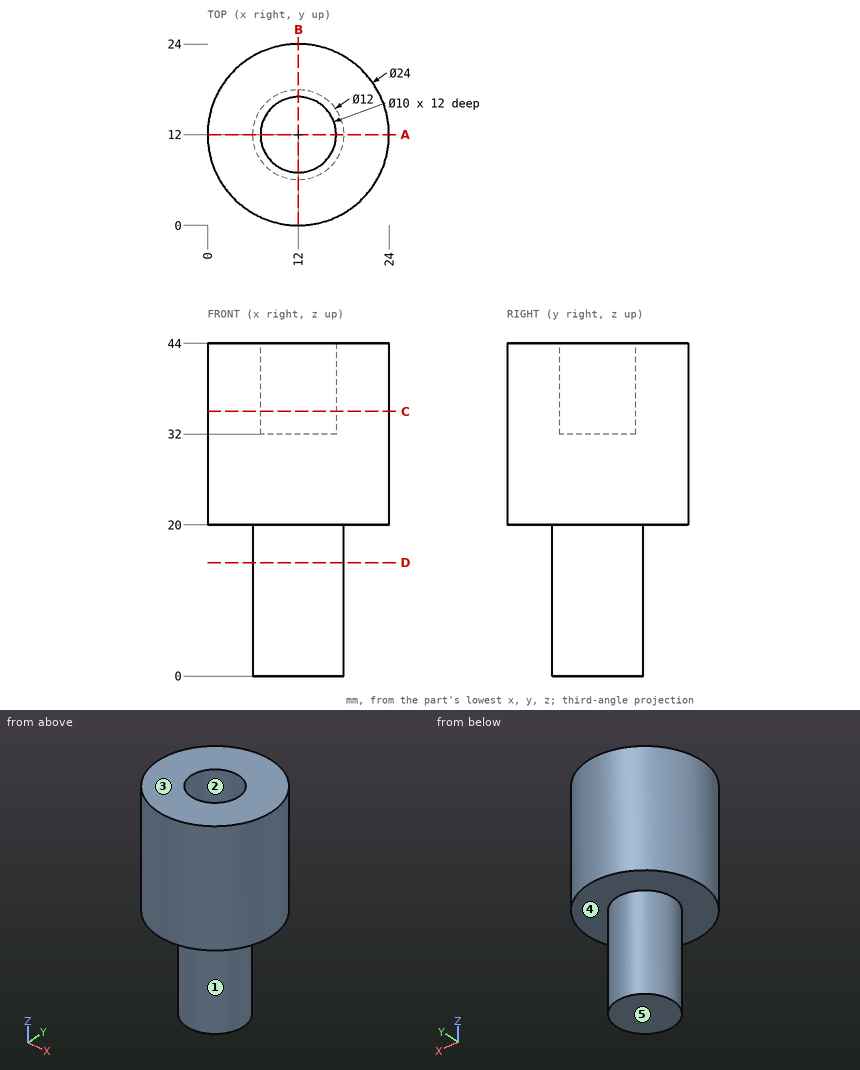
Design review of the part shown in the three views and the two pictorial views. Dimensions are in mm from the part's minimum x, y and z. A direction names the side the tool comes from. Round coordinates to 2 decimals unless told otherwise and drop trailing zeros. Write each loop counter-clockwise with the first axis right and the second up, starting at its lowest first coordinate (ties: lowest second). Pieces come first, ordered by that corner, then holes. Notation, with made-up numbers: M 59.25,70.25 L 112.25,70.25 A16 ccw 112.25,77.25 Z; hole C -2,30.5 d9. An arc over 180 degrees is marked long. Use a Markdown table: item, result. Add a question column.
Q1. We need section D-D, the plane z = 15. State the section outline as (x, y) points, plus the area to 3 significant figures.
Q2. Machinability: for the marked faces 4 and 5, which of the approach directions +Z, -Z, +X, -X, +Y, -Y give a long, thin tool a straight path to every point of the face, cutting with its end or side? Answer none if there is none.
Q3. To check wall thickness, follow line 1 (Y direction, x = 12, z = 38.75); line 2 (Z direction, x = 15.25, y = 12); line 3 (Z direction, x = 19, y = 18.25). State the ranges of each line that lie inside material, in increasing order.
Q4. Insertion check: pin 1 (12 mm diameter, centred on x = 3.5, z = 5, fed in from +Y); pin 2 (8 mm diameter, centred on x = 3, z = 39.5, fed in from +Y); pin 3 (5 mm diameter, centred on x = 5, z = 22, fed in from +Y). Each pin has a flat end and moves straight along its axis. Give the tip position at first contact, or say it passes through.
Q5. We need section A-A, the plane y = 12. State the section outline as (x, z) points, plus the area to 3 significant figures.
Q6. We need section C-C, the plane z = 35. State the section outline as (x, y) points.
Q7. The part is to be moulded in two halves that separate along Y. For the marked faces 1, 2 and 3, say which applies: pulls with the +Y half, pulls with the -Y half, needs draft (parallel to the pull), parting line crosses it, or undercut.
Findings below:
| question | item | result |
|---|---|---|
| 1 | outline | C 12,12 d12 |
| 1 | area | 113 mm² |
| 2 | face 4 | -Z |
| 2 | face 5 | -Z, +X, -X, +Y, -Y |
| 3 | line 1 | y = 0 to 7, 17 to 24 |
| 3 | line 2 | z = 0 to 32 |
| 3 | line 3 | z = 20 to 44 |
| 4 | pin 1 | stops at y = 17.45 |
| 4 | pin 2 | stops at y = 22.91 |
| 4 | pin 3 | stops at y = 23.12 |
| 5 | outline | M 0,20 L 6,20 L 6,0 L 18,0 L 18,20 L 24,20 L 24,44 L 17,44 L 17,32 L 7,32 L 7,44 L 0,44 Z |
| 5 | area | 696 mm² |
| 6 | outline | C 12,12 d24; hole C 12,12 d10 |
| 7 | face 1 | parting line crosses it |
| 7 | face 2 | undercut |
| 7 | face 3 | needs draft |
